Geometry check sheet. Reference: drawing and pictorial views, mm from the part's lowest x, y, z. Give positions to 0.01 mm unless a question says otherwise; leave off trailing zeros. Write each loop counter-clockwise with the first axis right and the second up, starting at its lowest first coordinate (ties: lowest second). Pieces come first, ordered by that corner, then holes. Notation, with made-up numbers: (-11.75, -27.5) - (37.25, -27.5) arc R17 cw to (37.25, -0.5) - close; hole circle Ø10 at (33.5, 42). An arc over 180 degrees is marked (long way). Write item = value, one per line. Start each with the question number.
(1) Section check D-D, the plane y = 24. Enter the section's corners in (x, z).
(2) Section check A-A, the plane x = 5.5. Enter the section's corners in (y, z), plus the area to 3 significant figures.
(3) Draft check along X on the marked faces 1 and 2. Enter one of: pulls with the +X half, pulls with the -X half, needs draft (parallel to the pull), parting line crosses it, or undercut.
(4) Thickness scan on L1, parallel to Y at x = 5.5, z = 2.7; L2, parallel to X at y = 24.5, z = 3.85; L3, parallel to Y at x = 21, z = 2.9. Record the ranges inside material, lowest first.
(5) Depth check by flat-ended pin: pin 1 Ø20.5 at (x, y) = (21, 24) entering from +Z. Enter the tip coordinate at first touch or a pass-through.
(6) Section check C-C, the plane z = 2.05. Enter the section's corners in (x, y), plus the area to 3 significant figures.
(7) Section check B-B, the plane y = 8.5. Enter the section's corners in (x, z).
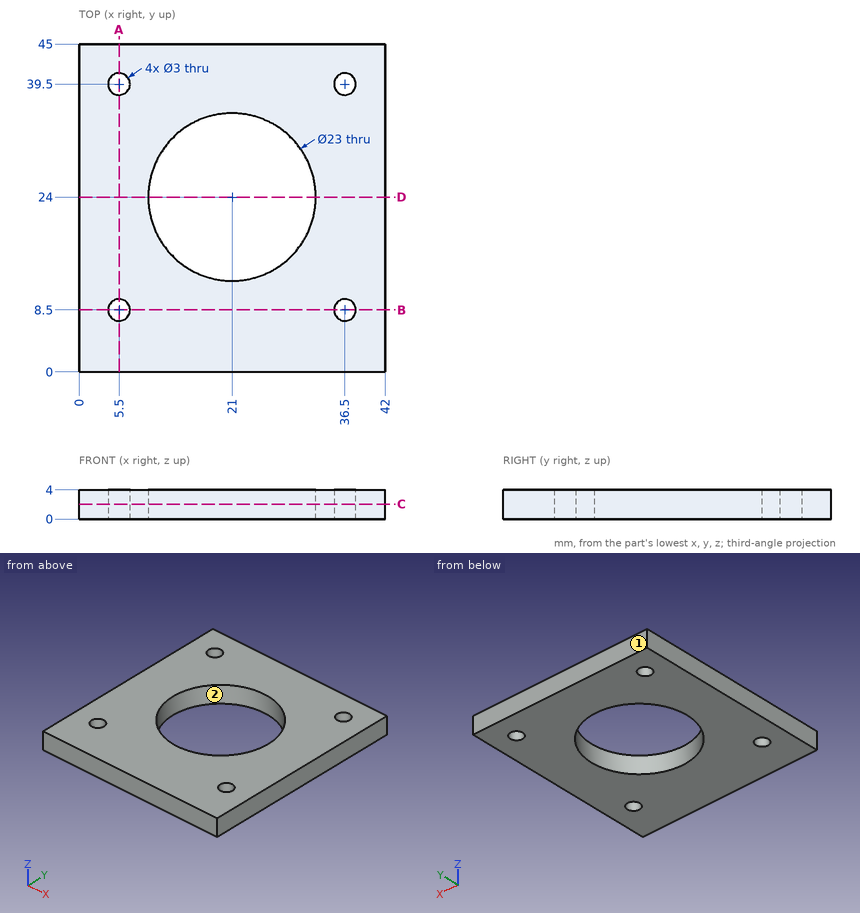
Model answer:
q1.outline = (0, 0) - (9.5, 0) - (9.5, 4) - (0, 4) - close; (32.5, 0) - (42, 0) - (42, 4) - (32.5, 4) - close
q2.outline = (0, 0) - (7, 0) - (7, 4) - (0, 4) - close; (10, 0) - (38, 0) - (38, 4) - (10, 4) - close; (41, 0) - (45, 0) - (45, 4) - (41, 4) - close
q2.area = 156 mm²
q3.face_1 = needs draft
q3.face_2 = undercut
q4.L1 = 0 to 7, 10 to 38, 41 to 45
q4.L2 = 0 to 9.51, 32.49 to 42
q4.L3 = 0 to 12.5, 35.5 to 45
q5.pin_1 = through
q6.outline = (0, 0) - (42, 0) - (42, 45) - (0, 45) - close; hole circle Ø3 at (5.5, 8.5); hole circle Ø3 at (5.5, 39.5); hole circle Ø23 at (21, 24); hole circle Ø3 at (36.5, 8.5); hole circle Ø3 at (36.5, 39.5)
q6.area = 1,450 mm²
q7.outline = (0, 0) - (4, 0) - (4, 4) - (0, 4) - close; (7, 0) - (35, 0) - (35, 4) - (7, 4) - close; (38, 0) - (42, 0) - (42, 4) - (38, 4) - close
